Read the model definition and answer for the solid it produces. Units are mm, in the model's axes. Face numbers are marked on the shaded views. A direction names the side the tool comes from. Give positions to 0.01 mm unless a question says otherwise; leave off trailing zeros. Loops run counter-clockwise (first coordinate to the right, second up) from the corner with the lowest first, then second, coordinate; pieces in that order, holes last. Notation, with made-up numbers: (-22.5, 21) - (-12.5, 21) arc R20 cw to (-12.5, 58) - close; hole circle Ø6 at (81.25, 74.5). An arc over 180 degrees is marked (long way). Use a Markdown table: item, result. Add a question column.
Item 1: A cutting plane is placed at B-B (y = -25.5). Determine the outline of the cut face in (x, z).
Item 2: Each of these flat-tipped pins is pushed along its axis until it touches: P1, Ø8, axis at y = 75, z = 28, coming from the -X side; P2, Ø9, axis at x = -51.5, y = 13.5, coming from the +Z side; P3, Ø1.5, axis at x = -52, y = -18.5, coming from the +Z side; P4, Ø2.5, axis at y = 94.82, z = 27, coming from the +X side. Where does it stop, or does it pass through?
Item 3: A cutting plane is placed at C-C (x = -44). Determine the outline of the cut face in (y, z).
Item 4: Consider probe 1 along Y at (x, z) = (-12, 13); probe 2 along X at (y, z) = (-10, 7.5); probe 3 along Y at (x, z) = (-49, 21). Determine where each line is inside the solid, lowest interval first. Write a range as [from, to].
Item 5: Which of the six approach directions +Z, -Z, +X, -X, +Y, -Y give full straight-line access (tool end or side, diameter ignored) to the marked faces 5, 6 and 7?
Item 6: For a pull along X with two mould halves and no side action, classify the marked faces 1, 2, 3 and 4 as +X half, -X half, draft (parallel to the pull), parting line (faces both ways), or undercut.
Item 7: A cutting plane is placed at A-A (z = 9). Give the number of separate pieces and of enclosed holes in the cut face, plus the area to 3 significant figures.
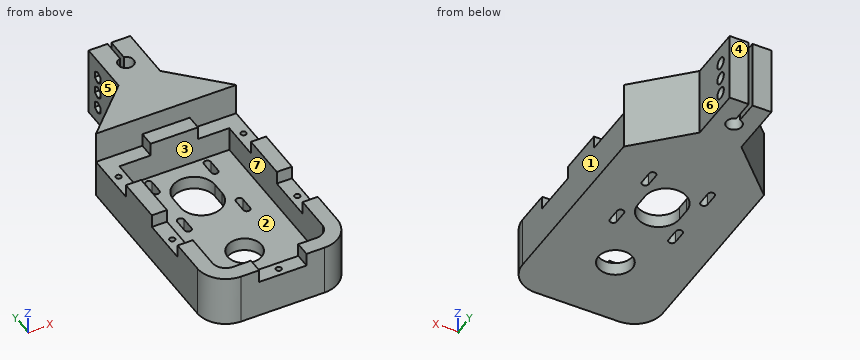
from build123d import *

# Parameters (mm, degrees)
CROQUIS2_R              = 9
SALIENTE_EXTRUIR1_DEPTH = 7
CROQUIS2_7_W            = 25
CROQUIS2_7_H            = 8
CROQUIS2_7_W_2          = 8
CROQUIS2_7_H_2          = 25
CROQUIS2_7_H_3          = 19
CROQUIS2_7_W_3          = 9.5
SALIENTE_EXTRUIR3_DEPTH = 27
CROQUIS2_12_W           = 8
CROQUIS2_12_H           = 25
CROQUIS2_12_W_2         = 25
CROQUIS2_12_H_2         = 8
SALIENTE_EXTRUIR4_DEPTH = 20
SALIENTE_EXTRUIR5_DEPTH = 37
CROQUIS4_R              = 1.475
CORTAR_EXTRUIR2_DEPTH   = 14
CROQUIS10_R             = 1.9
CORTAR_EXTRUIR3_DEPTH   = 22
CROQUIS11_R             = 3.1
CORTAR_EXTRUIR4_DEPTH   = 6
CORTAR_EXTRUIR5_DEPTH   = 6


with BuildPart() as part:
    # Croquis2 → Saliente-Extruir1 (new body)
    with BuildSketch(Plane.XY):
        with BuildLine():
            Line((-5.786620614, -56.183989891), (3.713379386, -56.183989891))
            ThreePointArc((3.713379386, -56.183989891), (8.663126854, -54.133737359), (10.713379386, -49.183989891))
            Line((10.713379386, -49.183989891), (10.713379386, -30.183989891))
            Line((10.713379386, -30.183989891), (10.713379386, -5.183989891))
            Line((10.713379386, -5.183989891), (10.713379386, 19.816010109))
            Line((10.713379386, 19.816010109), (10.713379386, 40.816010109))
            Line((10.713379386, 40.816010109), (-5.786620614, 40.816010109))
            Line((-5.786620614, 40.816010109), (-30.786620614, 40.816010109))
            Line((-30.786620614, 40.816010109), (-47.286620614, 40.816010109))
            Line((-47.286620614, 40.816010109), (-47.286620614, 19.816010109))
            Line((-47.286620614, 19.816010109), (-47.286620614, -5.183989891))
            Line((-47.286620614, -5.183989891), (-47.286620614, -30.183989891))
            Line((-47.286620614, -30.183989891), (-47.286620614, -49.183989891))
            ThreePointArc((-47.286620614, -49.183989891), (-45.236368082, -54.133737359), (-40.286620614, -56.183989891))
            Line((-40.286620614, -56.183989891), (-30.786620614, -56.183989891))
            Line((-30.786620614, -56.183989891), (-5.786620614, -56.183989891))
        make_face()
        with Locations((-18.286620614, -27.183989891)):
            Circle(CROQUIS2_R, mode=Mode.SUBTRACT)
        with BuildLine():
            ThreePointArc((-31.986620614, 6.205288522), (-33.786620614, 8.005288522), (-35.586620614, 6.205288522))
            Line((-35.586620614, 6.205288522), (-35.586620614, -0.794711478))
            ThreePointArc((-35.586620614, -0.794711478), (-33.786620614, -2.594711478), (-31.986620614, -0.794711478))
            Line((-31.986620614, -0.794711478), (-31.986620614, 6.205288522))
        make_face(mode=Mode.SUBTRACT)
        with BuildLine():
            ThreePointArc((-4.586620614, 30.205288522), (-2.786620614, 28.405288522), (-0.986620614, 30.205288522))
            Line((-0.986620614, 30.205288522), (-0.986620614, 37.205288522))
            ThreePointArc((-0.986620614, 37.205288522), (-2.786620614, 39.005288522), (-4.586620614, 37.205288522))
            Line((-4.586620614, 37.205288522), (-4.586620614, 30.205288522))
        make_face(mode=Mode.SUBTRACT)
        with BuildLine():
            ThreePointArc((-29.286620614, 14.705288522), (-18.286620614, 3.705288522), (-7.286620614, 14.705288522))
            Line((-7.286620614, 14.705288522), (-7.286620614, 21.705288522))
            ThreePointArc((-7.286620614, 21.705288522), (-18.286620614, 32.705288522), (-29.286620614, 21.705288522))
            Line((-29.286620614, 21.705288522), (-29.286620614, 14.705288522))
        make_face(mode=Mode.SUBTRACT)
        with BuildLine():
            Line((-0.986620614, 6.205288522), (-0.986620614, -0.794711478))
            ThreePointArc((-0.986620614, -0.794711478), (-2.786620614, -2.594711478), (-4.586620614, -0.794711478))
            Line((-4.586620614, -0.794711478), (-4.586620614, 6.205288522))
            ThreePointArc((-4.586620614, 6.205288522), (-2.786620614, 8.005288522), (-0.986620614, 6.205288522))
        make_face(mode=Mode.SUBTRACT)
        with BuildLine():
            Line((-35.586620614, 30.205288522), (-35.586620614, 37.205288522))
            ThreePointArc((-35.586620614, 37.205288522), (-33.786620614, 39.005288522), (-31.986620614, 37.205288522))
            Line((-31.986620614, 37.205288522), (-31.986620614, 30.205288522))
            ThreePointArc((-31.986620614, 30.205288522), (-33.786620614, 28.405288522), (-35.586620614, 30.205288522))
        make_face(mode=Mode.SUBTRACT)
    extrude(amount=SALIENTE_EXTRUIR1_DEPTH)

    # Croquis2_7 → Saliente-Extruir3 (add)
    with BuildSketch(Plane.XY):
        with Locations((-18.286620614, 44.816010109)):
            Rectangle(CROQUIS2_7_W, CROQUIS2_7_H)
        with Locations((-51.286620614, 7.316010109)):
            Rectangle(CROQUIS2_7_W_2, CROQUIS2_7_H_2)
        with Locations((-51.286620614, -39.683989891)):
            Rectangle(CROQUIS2_7_W_2, CROQUIS2_7_H_3)
        with BuildLine():
            ThreePointArc((-47.286620614, -49.183989891), (-45.236368082, -54.133737359), (-40.286620614, -56.183989891))
            Line((-40.286620614, -56.183989891), (-40.286620614, -64.183989891))
            ThreePointArc((-40.286620614, -64.183989891), (-50.893222332, -59.790591609), (-55.286620614, -49.183989891))
            Line((-55.286620614, -49.183989891), (-47.286620614, -49.183989891))
        make_face()
        with Locations((-35.536620614, -60.183989891)):
            Rectangle(CROQUIS2_7_W_3, CROQUIS2_7_H)
        with Locations((-1.036620614, -60.183989891)):
            Rectangle(CROQUIS2_7_W_3, CROQUIS2_7_H)
        with BuildLine():
            ThreePointArc((3.713379386, -56.183989891), (8.663126854, -54.133737359), (10.713379386, -49.183989891))
            Line((10.713379386, -49.183989891), (18.713379386, -49.183989891))
            ThreePointArc((18.713379386, -49.183989891), (14.319981104, -59.790591609), (3.713379386, -64.183989891))
            Line((3.713379386, -64.183989891), (3.713379386, -56.183989891))
        make_face()
        with Locations((14.713379386, -39.683989891)):
            Rectangle(CROQUIS2_7_W_2, CROQUIS2_7_H_3)
        with Locations((14.713379386, 7.316010109)):
            Rectangle(CROQUIS2_7_W_2, CROQUIS2_7_H_2)
    extrude(amount=SALIENTE_EXTRUIR3_DEPTH)

    # Croquis2_12 → Saliente-Extruir4 (add)
    with BuildSketch(Plane.XY):
        Polygon((10.713379386, 40.816010109), (-5.786620614, 40.816010109), (-5.786620614, 48.816010109), (18.713379386, 48.816010109), (18.713379386, 19.816010109), (10.713379386, 19.816010109), align=None)
        Polygon((-47.286620614, 19.816010109), (-47.286620614, 40.816010109), (-30.786620614, 40.816010109), (-30.786620614, 48.816010109), (-55.286620614, 48.816010109), (-55.286620614, 19.816010109), align=None)
        with Locations((-51.286620614, -17.683989891)):
            Rectangle(CROQUIS2_12_W, CROQUIS2_12_H)
        with Locations((14.713379386, -17.683989891)):
            Rectangle(CROQUIS2_12_W, CROQUIS2_12_H)
        with Locations((-18.286620614, -60.183989891)):
            Rectangle(CROQUIS2_12_W_2, CROQUIS2_12_H_2)
    extrude(amount=SALIENTE_EXTRUIR4_DEPTH)

    # Croquis2_14 → Saliente-Extruir5 (add)
    with BuildSketch(Plane.XY):
        with BuildLine():
            ThreePointArc((-19.286620614, 91.616010109), (-18.286620614, 83.539831039), (-17.286620614, 91.616010109))
            Line((-17.286620614, 91.616010109), (-17.286620614, 103.616010109))
            Line((-17.286620614, 103.616010109), (-7.286620614, 103.616010109))
            Line((-7.286620614, 103.616010109), (-7.286620614, 74.616010109))
            Line((-7.286620614, 74.616010109), (18.713379386, 48.816010109))
            Line((18.713379386, 48.816010109), (-5.786620614, 48.816010109))
            Line((-5.786620614, 48.816010109), (-30.786620614, 48.816010109))
            Line((-30.786620614, 48.816010109), (-55.286620614, 48.816010109))
            Line((-55.286620614, 48.816010109), (-29.286620614, 74.616010109))
            Line((-29.286620614, 74.616010109), (-29.286620614, 103.616010109))
            Line((-29.286620614, 103.616010109), (-19.286620614, 103.616010109))
            Line((-19.286620614, 103.616010109), (-19.286620614, 91.616010109))
        make_face()
    extrude(amount=SALIENTE_EXTRUIR5_DEPTH)

    # Croquis4 → Cortar-Extruir2 (cut)
    with BuildSketch(Plane.XY.offset(27)):
        with Locations((-51.286620614, 34.316010109)):
            Circle(CROQUIS4_R)
        with Locations((-51.286620614, -17.683989891)):
            Circle(CROQUIS4_R)
        with Locations((-18.286620614, -60.183989891)):
            Circle(CROQUIS4_R)
        with Locations((14.713379386, -17.683989891)):
            Circle(CROQUIS4_R)
        with Locations((14.713379386, 34.316010109)):
            Circle(CROQUIS4_R)
    extrude(amount=-CORTAR_EXTRUIR2_DEPTH, mode=Mode.SUBTRACT)

    # Croquis10 → Cortar-Extruir3 (cut)
    with BuildSketch(Plane(origin=(-7.286620614, 0, 0), x_dir=(0, 0, -1), z_dir=(1, 0, 0))):
        with Locations((-9, 94.816010109)):
            Circle(CROQUIS10_R)
        with Locations((-18, 94.816010109)):
            Circle(CROQUIS10_R)
        with Locations((-27, 94.816010109)):
            Circle(CROQUIS10_R)
    extrude(amount=-CORTAR_EXTRUIR3_DEPTH, mode=Mode.SUBTRACT)

    # Croquis11 → Cortar-Extruir4 (cut)
    with BuildSketch(Plane(origin=(-7.286620614, 0, 0), x_dir=(0, 0, -1), z_dir=(1, 0, 0))):
        with Locations((-27, 94.816010109)):
            Circle(CROQUIS11_R)
        with Locations((-18, 94.816010109)):
            Circle(CROQUIS11_R)
        with Locations((-9, 94.816010109)):
            Circle(CROQUIS11_R)
    extrude(amount=-CORTAR_EXTRUIR4_DEPTH, mode=Mode.SUBTRACT)

    # Croquis12 → Cortar-Extruir5 (cut)
    with BuildSketch(Plane.ZY.offset(29.286620614)):
        Polygon((21.233161507, 94.816010109), (19.616580754, 97.616010109), (16.383419246, 97.616010109), (14.766838493, 94.816010109), (16.383419246, 92.016010109), (19.616580754, 92.016010109), align=None)
        Polygon((12.233161507, 94.816010109), (10.616580754, 97.616010109), (7.383419246, 97.616010109), (5.766838493, 94.816010109), (7.383419246, 92.016010109), (10.616580754, 92.016010109), align=None)
        Polygon((30.233161507, 94.816010109), (28.616580754, 97.616010109), (25.383419246, 97.616010109), (23.766838493, 94.816010109), (25.383419246, 92.016010109), (28.616580754, 92.016010109), align=None)
    extrude(amount=-CORTAR_EXTRUIR5_DEPTH, mode=Mode.SUBTRACT)


solid = part.part
Geometry says:
| question | item | result |
|---|---|---|
| 1 | outline | (-55.29, 0) - (-27.13, 0) - (-27.13, 7) - (-47.29, 7) - (-47.29, 20) - (-55.29, 20) - close; (-9.45, 0) - (18.71, 0) - (18.71, 20) - (10.71, 20) - (10.71, 7) - (-9.45, 7) - close |
| 2 | P1 | x = -32.93 |
| 2 | P2 | z = 27 |
| 2 | P3 | z = 20 |
| 2 | P4 | through |
| 3 | outline | (-63.72, 0) - (60.02, 0) - (60.02, 37) - (48.82, 37) - (48.82, 20) - (40.82, 20) - (40.82, 7) - (-55.12, 7) - (-55.12, 27) - (-63.72, 27) - close |
| 4 | probe 1 | [-64.18, -56.18], [40.82, 103.62] |
| 4 | probe 2 | [-55.29, -47.29], [10.71, 18.71] |
| 4 | probe 3 | [-61.39, -30.18], [-5.18, 19.82], [48.82, 55.05] |
| 5 | face 5 | +Z, -Z, -X, +Y |
| 5 | face 6 | +Z, -Z, +X, +Y |
| 5 | face 7 | +Z |
| 6 | face 1 | +X half |
| 6 | face 2 | undercut |
| 6 | face 3 | undercut |
| 6 | face 4 | draft |
| 7 | separate pieces | 3 |
| 7 | enclosed holes | 1 |
| 7 | area | 4,360 mm² |
